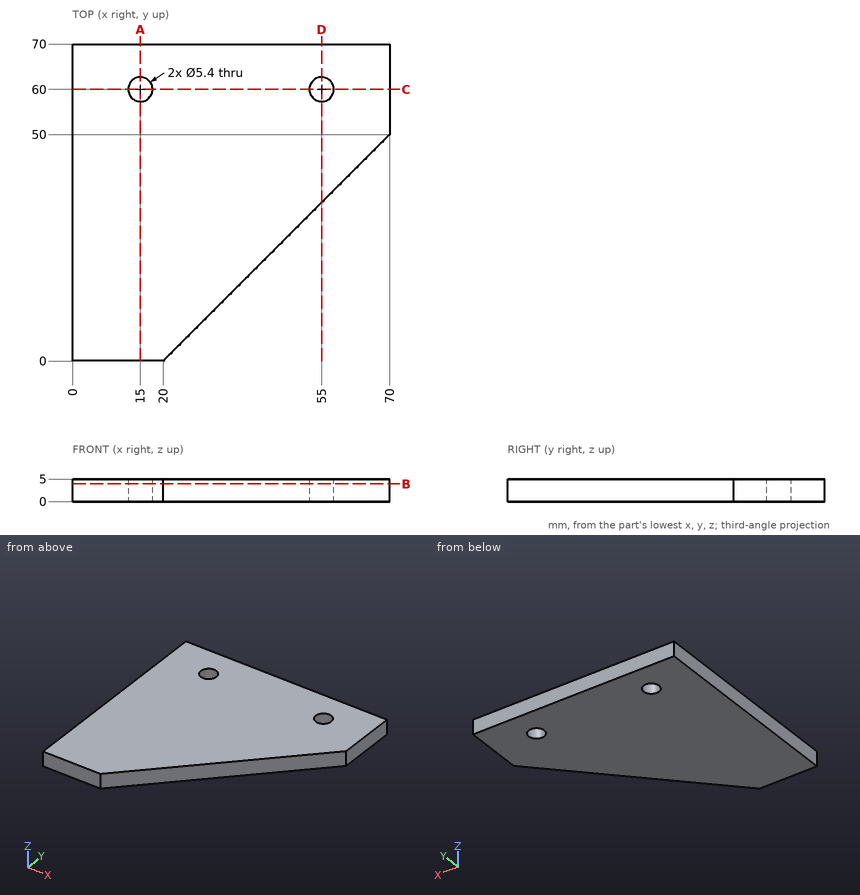
Can you work these out from the drawing? Everything is in mm from the part's minimum corner. Give positions to 0.01 mm unless a question says otherwise; leave off trailing zeros. Order: outer loops, then holes, each group sorted by start corner. A loop starts at its lowest first (then second) coordinate and runs counter-clockwise, first axis right, second up. Notation, with made-up numbers: M -9,54.5 L 38,54.5 A32 cw 38,90.5 Z; hole C -19,-35.75 d9. An arc over 180 degrees is marked long. One line per question, with ' | ' between items.
1. If I drill on line 1 (Y direction, x = 15, z = 1.6); line 2 (Y direction, x = 55, z = 3.4); line 3 (Y direction, x = 23, z = 4.05), over which ranges is the centre line in solid material (lowest first)?
Results:
line 1: 0 to 57.3, 62.7 to 70 | line 2: 35 to 57.3, 62.7 to 70 | line 3: 3 to 70
2. I want a section at D-D (x = 55). List the corners of the cut face in (y, z) for me, and give its area (3 significant figures).
Results:
outline: M 35,0 L 57.3,0 L 57.3,5 L 35,5 Z; M 62.7,0 L 70,0 L 70,5 L 62.7,5 Z | area: 148 mm²
3. I want a section at A-A (x = 15). List the corners of the cut face in (y, z) for me.
Results:
outline: M 0,0 L 57.3,0 L 57.3,5 L 0,5 Z; M 62.7,0 L 70,0 L 70,5 L 62.7,5 Z
4. I want a section at B-B (z = 3.9). List the corners of the cut face in (x, y) for me, and give its area (3 significant figures).
Results:
outline: M 0,0 L 20,0 L 70,50 L 70,70 L 0,70 Z; hole C 15,60 d5.4; hole C 55,60 d5.4 | area: 3,600 mm²
5. I'm going to push a flat-ended pin straight in: pin 1 (1.5 mm diameter, centred on y = 26.5, z = 2, fed in from -X). Where does the tip first touch, or does it pass through?
Results:
pin 1: x = 0
6. I want a section at C-C (y = 60). List the corners of the cut face in (x, z) for me, and give its area (3 significant figures).
Results:
outline: M 0,0 L 12.3,0 L 12.3,5 L 0,5 Z; M 17.7,0 L 52.3,0 L 52.3,5 L 17.7,5 Z; M 57.7,0 L 70,0 L 70,5 L 57.7,5 Z | area: 296 mm²
